from build123d import *

# Parameters (mm, degrees)
F1_DEPTH = 25
F2_R     = 1


with BuildPart() as f1:
    # F0 (on Right) → F1 (new body)
    with BuildSketch(Plane.YZ):
        Polygon((-25, 0), (0, 0), (0, 30.977491), (-25, 10), align=None)
    extrude(amount=F1_DEPTH)

    # F2
    f2_edges = [f1.edges().sort_by_distance(p)[0] for p in [
        (12.5, 0, 0),
        (12.5, 0, 30.977491),
        (0, 0, 15.488745),
        (25, 0, 15.488745),
        (12.5, -25, 10),
        (0, -12.5, 20.488745),
        (25, -12.5, 20.488745),
        (12.5, -25, 0),
        (0, -25, 5),
        (25, -25, 5),
        (25, -12.5, 0),
        (0, -12.5, 0),
    ]]
    fillet(f2_edges, radius=F2_R)


solid = f1.part
Geometry: final body of the model. Coordinates: model frame, mm. Give positions to 0.01 mm unless a question says otherwise; leave off trailing zeros. Loops run counter-clockwise (first coordinate to the right, second up) from the corner with the lowest first, then second, coordinate; pieces in that order, holes last. Notation, with made-up numbers: M 61.5,72.5 L 92.5,72.5 A32 cw 92.5,102.5 Z; hole C 5.5,74.5 d4. An arc over 180 degrees is marked long. Put each result on its own line as item: value. Start each with the question number.
1) Ray query, line 1 along Z through (x, y) = (19.5, -3); line 2 along Y through (x, z) = (23.75, 24.25); line 3 along Y through (x, z) = (22.25, 13). Return the intervals inside material, ascending.
2) Contact query for flat-ended pins moving along their axis: pin 1 (1.5 mm diameter, centred on x = 18.5, y = -15.5, fed in from +Z); pin 2 (1 mm diameter, centred on y = -6, z = 4, fed in from -X); pin 3 (3 mm diameter, centred on x = 18.5, y = -13, fed in from +Z). Output: stop coordinate, or through.
3) Cut plane A-A (x = 8.75). Output: boundary loops of the cut face in (y, z), then the cut area to 3 significant figures.
Verdict:
1. line 1: 0 to 28.46
1. line 2: -8.02 to 0
1. line 3: -21.42 to 0
2. pin 1: z = 18.6
2. pin 2: x = 0
2. pin 3: z = 21.33
3. outline: M -25,1 A1 ccw -24,0 L -1,0 A1 ccw 0,1 L 0,28.83 A1 ccw -1.64,29.6 L -24.64,10.3 A1 ccw -25,9.53 Z
3. area: 511 mm2
